from build123d import *

# Parameters (mm, degrees)
BOSS_EXTRUDE1_DEPTH     = 2
CUT_EXTRUDE2_DEPTH      = 88.82368701
CUT_EXTRUDE2_DEPTH_BACK = 88.82368701
SKETCH2_R               = 1.5
CUT_EXTRUDE7_START      = 2
SKETCH3_W               = 10
SKETCH3_H               = 12.1
SKETCH3_W_2             = 11
SKETCH3_H_2             = 9.5
CUT_EXTRUDE7_DEPTH      = 0.4
BOSS_EXTRUDE2_DEPTH     = 3
LPATTERN1_COUNT         = 3
LPATTERN1_PITCH         = 3
SKETCH5_W               = 0.724136619
SKETCH5_H               = 0.689653923
BOSS_EXTRUDE4_DEPTH     = 8
BOSS_EXTRUDE5_DEPTH     = 3
LPATTERN3_COUNT         = 3
LPATTERN3_PITCH         = 3
SKETCH8_W               = 0.829728978
SKETCH8_H               = 0.730951718
BOSS_EXTRUDE6_DEPTH     = 8
SKETCH9_W               = 6.486986995
SKETCH9_H               = 5.963842883
BOSS_EXTRUDE7_DEPTH     = 2
SKETCH11_R              = 1.680495579
BOSS_EXTRUDE8_DEPTH     = 1
BOSS_EXTRUDE9_DEPTH     = 1
BOSS_EXTRUDE10_DEPTH    = 3
BOSS_EXTRUDE11_DEPTH    = 1
BOSS_EXTRUDE12_DEPTH    = 3
SKETCH16_R              = 3
BOSS_EXTRUDE13_DEPTH    = 3
FILLET1_R               = 0.3


with BuildPart() as part:
    # Sketch1 → Boss-Extrude1 (new body)
    with BuildSketch(Plane(origin=(0, 0, 0), x_dir=(1, 0, 0), z_dir=(0, 1, 0))):
        Polygon((0, 0), (66, 0), (66, 4), (70, 7.100943302), (70, 37.450193791), (66, 41), (66, 53), (0, 53), align=None)
    extrude(amount=BOSS_EXTRUDE1_DEPTH)

    # Sketch2 → Cut-Extrude2 (cut, two sides: drawn at the far end of the back side and taken through both)
    with BuildSketch(Plane(origin=(0, 0, 0), x_dir=(1, 0, 0), z_dir=(0, 1, 0)).offset(-CUT_EXTRUDE2_DEPTH_BACK)):
        with Locations(Location((68, 35.450193791, 0), (0, 0, 270))):
            Circle(SKETCH2_R)
        with Locations(Location((68, 9.100943302, 0), (0, 0, 270))):
            Circle(SKETCH2_R)
        with Locations(Location((13.3, 2, 0), (0, 0, 270))):
            Circle(SKETCH2_R)
        with Locations(Location((13.3, 51, 0), (0, 0, 270))):
            Circle(SKETCH2_R)
    extrude(amount=CUT_EXTRUDE2_DEPTH + CUT_EXTRUDE2_DEPTH_BACK, mode=Mode.SUBTRACT)

    # Sketch3 → Cut-Extrude7 (cut)
    with BuildSketch(Plane(origin=(0, 0, 0), x_dir=(1, 0, 0), z_dir=(0, 1, 0)).offset(CUT_EXTRUDE7_START)):
        with Locations((5, 38.95)):
            Rectangle(SKETCH3_W, SKETCH3_H)
        with Locations((5.5, 9.75)):
            Rectangle(SKETCH3_W_2, SKETCH3_H_2)
    extrude(amount=-CUT_EXTRUDE7_DEPTH, mode=Mode.SUBTRACT)

    # Sketch4 → Boss-Extrude2 (add)
    with BuildSketch(Plane(origin=(0, 2, 0), x_dir=(1, 0, 0), z_dir=(0, 1, 0))):
        Polygon((63.879895434, 30.5), (63.379895434, 30), (63.379895434, 28), (63.879895434, 27.5), (67.879895434, 27.5), (68.379895434, 28), (68.379895434, 30), (67.879895434, 30.5), align=None)
    boss_extrude2 = extrude(amount=BOSS_EXTRUDE2_DEPTH)

    # LPattern1: Boss-Extrude2 ×3
    with Locations(*[(0, 0, i * LPATTERN1_PITCH) for i in range(1, LPATTERN1_COUNT)]):
        add(boss_extrude2)

    # Sketch5 → Boss-Extrude4 (add)
    with BuildSketch(Plane(origin=(0, 5, 0), x_dir=(1, 0, 0), z_dir=(0, 1, 0))):
        with Locations((64.716683918, 28.923857239)):
            Rectangle(SKETCH5_W, SKETCH5_H)
        with Locations((67.04310695, 28.923857239)):
            Rectangle(SKETCH5_W, SKETCH5_H)
        with Locations((67.04310695, 26.076142762)):
            Rectangle(SKETCH5_W, SKETCH5_H)
        with Locations((64.716683918, 26.076142762)):
            Rectangle(SKETCH5_W, SKETCH5_H)
        with Locations((67.04310695, 22.923857239)):
            Rectangle(SKETCH5_W, SKETCH5_H)
        with Locations((64.716683918, 22.923857239)):
            Rectangle(SKETCH5_W, SKETCH5_H)
    extrude(amount=BOSS_EXTRUDE4_DEPTH)

    # Sketch6 → Boss-Extrude5 (add)
    with BuildSketch(Plane(origin=(0, 2, 0), x_dir=(1, 0, 0), z_dir=(0, 1, 0))):
        Polygon((17.282939777, 51), (19.282939777, 51), (19.782939777, 50.5), (19.782939777, 46.5), (19.282939777, 46), (17.282939777, 46), (16.782939777, 46.5), (16.782939777, 50.5), align=None)
    boss_extrude5 = extrude(amount=BOSS_EXTRUDE5_DEPTH)

    # LPattern3: Boss-Extrude5 ×3
    with Locations(*[(i * LPATTERN3_PITCH, 0, 0) for i in range(1, LPATTERN3_COUNT)]):
        add(boss_extrude5)

    # Sketch8 → Boss-Extrude6 (add)
    with BuildSketch(Plane(origin=(0, 5, 0), x_dir=(1, 0, 0), z_dir=(0, 1, 0))):
        with Locations((21.321404848, 49.61932377)):
            Rectangle(SKETCH8_W, SKETCH8_H)
        with Locations((18.244474705, 49.61932377)):
            Rectangle(SKETCH8_W, SKETCH8_H)
        with Locations((24.244474705, 49.61932377)):
            Rectangle(SKETCH8_W, SKETCH8_H)
        with Locations((24.244474705, 47.38067623)):
            Rectangle(SKETCH8_W, SKETCH8_H)
        with Locations((21.321404848, 47.38067623)):
            Rectangle(SKETCH8_W, SKETCH8_H)
        with Locations((18.244474705, 47.38067623)):
            Rectangle(SKETCH8_W, SKETCH8_H)
    extrude(amount=BOSS_EXTRUDE6_DEPTH)

    # Sketch9 → Boss-Extrude7 (add)
    with BuildSketch(Plane(origin=(0, 2, 0), x_dir=(1, 0, 0), z_dir=(0, 1, 0))):
        with Locations((54.045911219, 24.481921441)):
            Rectangle(SKETCH9_W, SKETCH9_H)
    extrude(amount=BOSS_EXTRUDE7_DEPTH)

    # Sketch11 → Boss-Extrude8 (add)
    with BuildSketch(Plane(origin=(0, 4, 0), x_dir=(1, 0, 0), z_dir=(0, 1, 0))):
        with Locations(Location((54.04591122, 24.481921441, 0), (0, 0, 270))):
            Circle(SKETCH11_R)
    extrude(amount=BOSS_EXTRUDE8_DEPTH)

    # Sketch12 → Boss-Extrude9 (add)
    with BuildSketch(Plane(origin=(0, 2, 0), x_dir=(1, 0, 0), z_dir=(0, 1, 0))):
        with BuildLine():
            Line((36.85972443, 24.919811949), (44.85972443, 24.919811949))
            ThreePointArc((44.85972443, 24.919811949), (46.85972443, 22.919811949), (44.85972443, 20.919811949))
            Line((44.85972443, 20.919811949), (36.85972443, 20.919811949))
            ThreePointArc((36.85972443, 20.919811949), (34.85972443, 22.919811949), (36.85972443, 24.919811949))
        make_face()
    extrude(amount=BOSS_EXTRUDE9_DEPTH)

    # Sketch13 → Boss-Extrude10 (add)
    with BuildSketch(Plane(origin=(0, 3, 0), x_dir=(1, 0, 0), z_dir=(0, 1, 0))):
        with BuildLine():
            Line((44.85972443, 24.419811949), (36.85972443, 24.419811949))
            ThreePointArc((36.85972443, 24.419811949), (35.35972443, 22.919811949), (36.85972443, 21.419811949))
            Line((36.85972443, 21.419811949), (44.85972443, 21.419811949))
            ThreePointArc((44.85972443, 21.419811949), (46.35972443, 22.919811949), (44.85972443, 24.419811949))
        make_face()
    extrude(amount=BOSS_EXTRUDE10_DEPTH)

    # Sketch14 → Boss-Extrude11 (add)
    with BuildSketch(Plane(origin=(0, 2, 0), x_dir=(1, 0, 0), z_dir=(0, 1, 0))):
        with BuildLine():
            Line((16.059725168, 34.595333511), (24.059725168, 34.595333511))
            ThreePointArc((24.059725168, 34.595333511), (26.059725168, 32.595333511), (24.059725168, 30.595333511))
            Line((24.059725168, 30.595333511), (16.059725168, 30.595333511))
            ThreePointArc((16.059725168, 30.595333511), (14.059725168, 32.595333511), (16.059725168, 34.595333511))
        make_face()
    extrude(amount=BOSS_EXTRUDE11_DEPTH)

    # Sketch15 → Boss-Extrude12 (add)
    with BuildSketch(Plane(origin=(0, 3, 0), x_dir=(1, 0, 0), z_dir=(0, 1, 0))):
        with BuildLine():
            Line((16.059725168, 31.095333511), (24.059725168, 31.095333511))
            ThreePointArc((24.059725168, 31.095333511), (25.559725168, 32.595333511), (24.059725168, 34.095333511))
            Line((24.059725168, 34.095333511), (16.059725168, 34.095333511))
            ThreePointArc((16.059725168, 34.095333511), (14.559725168, 32.595333511), (16.059725168, 31.095333511))
        make_face()
    extrude(amount=BOSS_EXTRUDE12_DEPTH)

    # Sketch16 → Boss-Extrude13 (add)
    with BuildSketch(Plane(origin=(0, 2, 0), x_dir=(1, 0, 0), z_dir=(0, 1, 0))):
        with Locations(Location((21.969175252, 4, 0), (0, 0, 270))):
            Circle(SKETCH16_R)
        with Locations(Location((30.025126654, 4, 0), (0, 0, 270))):
            Circle(SKETCH16_R)
    extrude(amount=BOSS_EXTRUDE13_DEPTH)

    # Fillet1
    fillet1_edges = [part.edges().sort_by_distance(p)[0] for p in [
        (21.969175252, 5, -7),
        (30.025126654, 5, -7),
    ]]
    fillet(fillet1_edges, radius=FILLET1_R)


solid = part.part
Can you work these out from the model? Positions are in its coordinate system, mm. A direction names the side the tool comes from. Round coordinates to 2 decimals unless told otherwise and drop trailing zeros. Order: outer loops, then holes, each group sorted by start corner. A loop starts at its lowest first (then second) coordinate and runs counter-clockwise, first axis right, second up. Notation, with made-up numbers: M 59,-9.5 L 90,-9.5 A14 cw 90,11.5 Z; hole C -9,38.25 d3. An arc over 180 degrees is marked long. Use a Markdown table: item, result.
1) Imagine slicing it at B-B (z = -48.5). List the corners of the cut face in (x, y) for me.
Geometry says:
| item | result |
|---|---|
| outline | M 0,0 L 66,0 L 66,2 L 25.78,2 L 25.78,5 L 16.78,5 L 16.78,2 L 0,2 Z |
2) I'm going to push flat-ended pins straight in: P1, Ø1, axis at y = 4, z = -25.5, coming from the -X side; P2, Ø1, axis at y = 3, z = -26, coming from the +X side; P3, Ø2, axis at x = 23.5, y = 11, coming from the -Z side. Where does each tip first touch, or does it pass through?
Geometry says:
| item | result |
|---|---|
| P1 | stops at x = 50.8 |
| P2 | stops at x = 68.38 |
| P3 | stops at z = -49.98 |
3) Imagine slicing it at C-C (y = 11.5). Give the number of separate pieces and of enclosed holes in the cut face, then the cut area to 3 significant figures.
Geometry says:
| item | result |
|---|---|
| separate pieces | 12 |
| enclosed holes | 0 |
| area | 6.64 mm² |
4) Imagine slicing it at D-D (x = 58). List the corners of the cut face in (y, z) for me, then the cut area to 3 significant figures.
Geometry says:
| item | result |
|---|---|
| outline | M 0,-53 L 2,-53 L 2,0 L 0,0 Z |
| area | 106 mm² |
5) Imagine slicing it at A-A (x = 13.3). List the corners of the cut face in (y, z) for me.
Geometry says:
| item | result |
|---|---|
| outline | M 0,-53 L 2,-53 L 2,-52.5 L 0,-52.5 Z; M 0,-49.5 L 2,-49.5 L 2,-3.5 L 0,-3.5 Z; M 0,-0.5 L 2,-0.5 L 2,0 L 0,0 Z |
6) On a 3-axis mill with a long thin cutter (end or side, diameter ignored), from which of +Z, -Z, +X, -X, +Y, -Y can I reach the whole of each face in a straight line? I mean faces 5 (the face through (46.36, 4.48, -22.89)), 6 (the face through (18, 3, -51)), 7 (the face through (16.783, 3, -48)), 8 (the face through (54, 5, -25)), 9 (the face through (5, 1.6, -39)). Say none if no direction works.
Geometry says:
| item | result |
|---|---|
| face 5 | +Y |
| face 6 | -Z, +X, -X, +Y |
| face 7 | -Z, -X, +Y |
| face 8 | +Z, -Z, +Y |
| face 9 | -X, +Y |
7) If I drill on line 1 along Z through (x, y) = (68, 0.85); line 2 along X through (y, z) = (0.75, -51); line 3 along Z through (x, y) = (13.3, 0.75), over which ranges is the centre line in solid material (lowest first)?
Geometry says:
| item | result |
|---|---|
| line 1 | z = -39.23 to -36.95, -33.95 to -10.6, -7.6 to -5.55 |
| line 2 | x = 0 to 11.8, 14.8 to 66 |
| line 3 | z = -53 to -52.5, -49.5 to -3.5, -0.5 to 0 |
8) If we mould it in two halves opening along X, with no side actions, what happens to faces 1 (the face through (63.38, 3, -23)), 2 (the face through (14.06, 2.49, -32.55)), 3 (the face through (70, 1, -22)), 4 (the face through (57.289, 3, -24))? For each: +X half, -X half, draft (parallel to the pull), parting line (faces both ways), or undercut.
Geometry says:
| item | result |
|---|---|
| face 1 | undercut |
| face 2 | -X half |
| face 3 | +X half |
| face 4 | undercut |
